Check sheet for the drawn part. Datum: minimum x, y, z corner. Units: mm. A direction names the side the tool comes from. Give positions to 0.01 mm unless a question says otherwise; leave off trailing zeros. Order: outer loops, then holes, each group sorted by start corner. A loop starts at its lowest first (then second) coordinate and runs counter-clockwise, first axis right, second up. Notation, with made-up numbers: M 27,75.5 L 74,75.5 A26 cw 74,100.5 Z; hole C 28.5,36 d2. An arc over 180 degrees is marked long. Put each result on its own line as item: value. Start each with the question number.
Q1. Mould release check, pull along Z, two halves, no side actions. Record for the marked faces 1, 2 and 3: +Z half, -Z half, draft (parallel to the pull), parting line (faces both ways), or undercut.
Q2. Access from +Z, -Z, +X, -X, +Y, -Y to the whole of each face (thin tool, end or side, straight path). Record for the marked faces 4 and 5.
Q3. Section check C-C on x = 9.4. Record the cut outline in (y, z), then the cut area to 3 significant figures.
Q4. Go/stop test with flat-tipped pins: pin 1 (3 mm diameter, centred on y = 3.5, z = 10, fed in from -X); pin 2 (3 mm diameter, centred on x = 9.4, z = 10, fed in from -Y); pin 3 (2 mm diameter, centred on x = 15.5, z = 11, fed in from +Y). Record where each tip stops, or that it passes through.
Q5. Material ranges on L1, parallel to Z at x = 22.7, y = 13; L2, parallel to Y at x = 23.5, z = 14; L3, parallel to Z at x = 9.4, y = 0.95, recorded low to high.
Q6. Section check A-A on y = 13. Record the cut outline in (x, z).
Q7. Section check B-B on z = 10. Record the cut outline in (x, y), then the cut area to 3 significant figures.
Q8. Section check D-D on x = 22.25. Record the cut outline in (y, z).
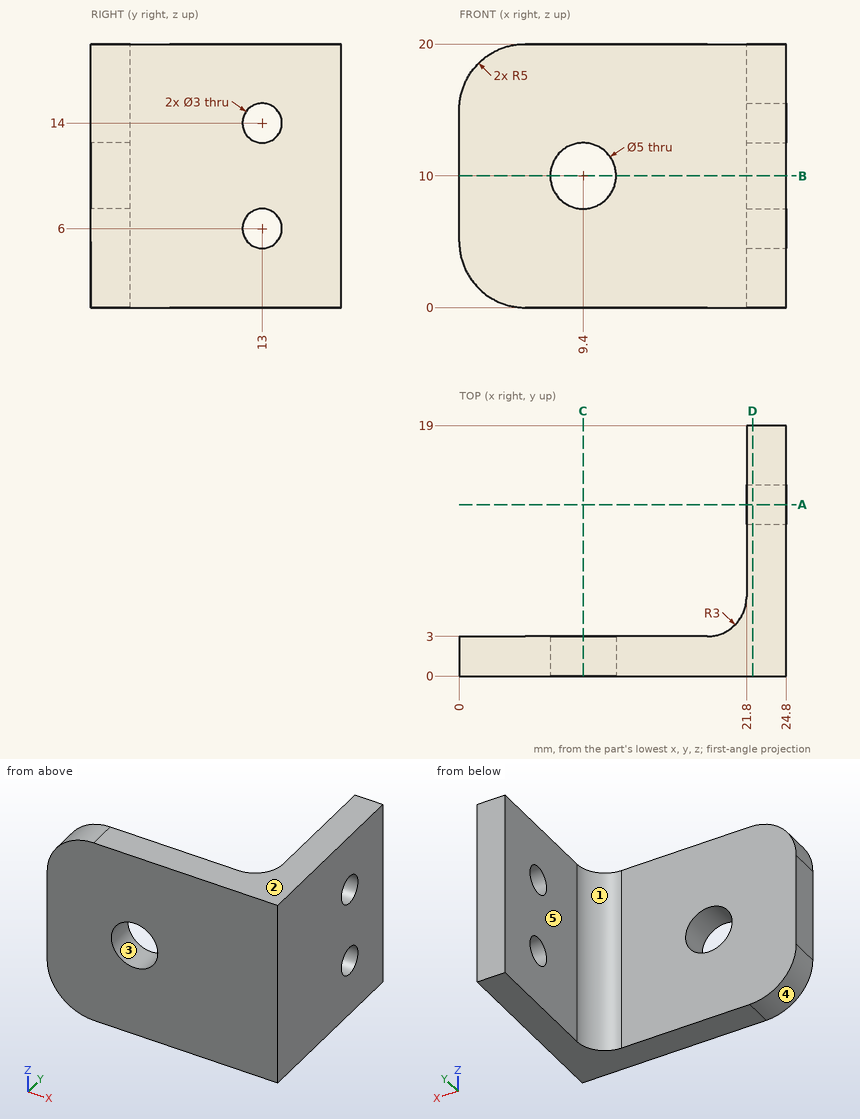
Results found:
1. face 1: draft
1. face 2: +Z half
1. face 3: undercut
2. face 4: -Z, -X, +Y, -Y
2. face 5: +Z, -Z, -X, +Y
3. outline: M 0,0 L 3,0 L 3,7.5 L 0,7.5 Z; M 0,12.5 L 3,12.5 L 3,20 L 0,20 Z
3. area: 45.0 mm^2
4. pin 1: stops at x = 0
4. pin 2: passes through
4. pin 3: stops at y = 3
5. L1: z = 0 to 4.5, 7.5 to 12.5, 15.5 to 20
5. L2: y = 0 to 11.5, 14.5 to 19
5. L3: z = 0 to 7.5, 12.5 to 20
6. outline: M 21.8,0 L 24.8,0 L 24.8,4.5 L 21.8,4.5 Z; M 21.8,7.5 L 24.8,7.5 L 24.8,12.5 L 21.8,12.5 Z; M 21.8,15.5 L 24.8,15.5 L 24.8,20 L 21.8,20 Z
7. outline: M 0,0 L 6.9,0 L 6.9,3 L 0,3 Z; M 11.9,0 L 24.8,0 L 24.8,19 L 21.8,19 L 21.8,6 A3 cw 18.8,3 L 11.9,3 Z
7. area: 109 mm^2
8. outline: M 0,0 L 19,0 L 19,20 L 0,20 Z; hole C 13,6 d3; hole C 13,14 d3
